Can you work these out from the model? Positions are in its coordinate system, mm. A direction names the side the tool comes from. Give positions to 0.01 mm unless a question says otherwise; leave off trailing zeros. Order: outer loops, then holes, each group sorted by start corner. A loop starts at its lowest first (then second) coordinate and runs counter-clockwise, first axis right, second up. Notation, with made-up numbers: M -15.5,33 L 21.5,33 A18 cw 21.5,60 Z; hole C 3.5,88 d10. An arc over 180 degrees is marked long. Write each question's results on one line, items separated by ' | '.
from build123d import *

# Parameters (mm, degrees)
EXTRUDE1_DEPTH              = 342.9
SKETCH2_R                   = 1.58758
SKETCH2_R_2                 = 4.826
EXTRUDE2_DEPTH              = 25
F_1_4_0_25_DIAMETER_HOLE1_D = 6.35
LPATTERN1_COUNT             = 27
LPATTERN1_PITCH             = 25.4


with BuildPart() as part:
    # Sketch1 → Extrude1 (new body, symmetric)
    with BuildSketch(Plane(origin=(0, 0, 0), x_dir=(1, 0, 0), z_dir=(0, 1, 0))):
        with BuildLine():
            Line((-12.7, 0), (-12.7, 22.225))
            ThreePointArc((-12.7, 22.225), (-11.77006403, 24.47006403), (-9.525, 25.4))
            Line((-9.525, 25.4), (9.525, 25.4))
            ThreePointArc((9.525, 25.4), (11.77006403, 24.47006403), (12.7, 22.225))
            Line((12.7, 22.225), (12.7, 0))
            Line((12.7, 0), (15.875, 0))
            Line((15.875, 0), (15.875, 22.225))
            ThreePointArc((15.875, 22.225), (14.015128061, 26.715128061), (9.525, 28.575))
            Line((9.525, 28.575), (-9.525, 28.575))
            ThreePointArc((-9.525, 28.575), (-14.015128061, 26.715128061), (-15.875, 22.225))
            Line((-15.875, 22.225), (-15.875, 0))
            Line((-15.875, 0), (-12.7, 0))
        make_face()
    extrude(amount=EXTRUDE1_DEPTH, both=True)

    # Sketch2 → Extrude2 (cut)
    with BuildSketch(Plane(origin=(0, 0, -28.575), x_dir=(-1, 0, 0), z_dir=(0, 0, -1))):
        with Locations((0, 342.9)):
            Circle(SKETCH2_R)
        with Locations((-1.905, 209.55)):
            Circle(SKETCH2_R_2)
        with Locations((-1.905, 184.15)):
            Circle(SKETCH2_R_2)
        with Locations((-1.905, -6.35)):
            Circle(SKETCH2_R_2)
        with Locations((1.905, 101.6)):
            Circle(SKETCH2_R_2)
        with Locations((-1.905, -260.35)):
            Circle(SKETCH2_R_2)
        with Locations((-1.905, -234.95)):
            Circle(SKETCH2_R_2)
        with Locations((-1.905, 19.05)):
            Circle(SKETCH2_R_2)
    extrude(amount=-EXTRUDE2_DEPTH, mode=Mode.SUBTRACT)

    # 1/4 (0.25) Diameter Hole1 (through all)
    with Locations(Plane.ZY.offset(15.875)):
        with Locations((-12.7, 330.2)):
            f_1_4_0_25_diameter_hole1 = Hole(F_1_4_0_25_DIAMETER_HOLE1_D / 2)

    # LPattern1: 1/4 (0.25) Diameter Hole1 ×27
    with Locations(*[(0, -i * LPATTERN1_PITCH, 0) for i in range(1, LPATTERN1_COUNT)]):
        add(f_1_4_0_25_diameter_hole1, mode=Mode.SUBTRACT)


solid = part.part
(1) Will these pins go through, and if not, where does the flat tip stop? P1, Ø7.5, axis at x = 1.905, y = -6.35, coming from the +Z side; P2, Ø5, axis at y = -49.5, z = -25.5, coming from the -X side.
Data:
P1: passes through | P2: stops at x = -15.83
(2) Imagine slicing it at A-A, the plane y = -294. Write out the boundary of the cut face in (x, z) (3 decimals), plus the area to 3 significant figures.
Data:
outline: M -15.875,-22.225 A6.35 ccw -9.525,-28.575 L 9.525,-28.575 A6.35 ccw 15.875,-22.225 L 15.875,0 L 12.7,0 L 12.7,-22.225 A3.175 cw 9.525,-25.4 L -9.525,-25.4 A3.175 cw -12.7,-22.225 L -12.7,0 L -15.875,0 Z | area: 249 mm2
(3) For faces 5 (the face through (-12.7, 5, -11)), 6 (the face through (0, 5, -28.575)), which set-ups out of +Z, -Z, +X, -X, +Y, -Y let a thin tool reach every point of the face, with its end or its side?
Data:
face 5: +Z, +Y, -Y | face 6: -Z, +X, -X, +Y, -Y
(4) We'd pull the mould along X, two halves only. Please class faces 1 (the face through (13, 342.9, -16)), 2 (the face through (15.875, 5, -11)), 3 (the face through (-15.875, 5, -11)), 4 (the face through (12.7, 5, -11)): +X half, -X half, draft (parallel to the pull), parting line (faces both ways), or undercut.
Data:
face 1: draft | face 2: +X half | face 3: -X half | face 4: undercut
(5) I need wall thicknesses on L1, parallel to X at y = 140.5, z = -12.75 (3 decimals); L2, parallel to Z at x = 15, y = -279; L3, parallel to Z at x = -0.5, y = -135.5 (3 decimals). Which ranges of each line are inside material? Lowest first, please. Write a range as from..to.
Data:
L1: x = -15.875..-12.7, 12.7..15.875 | L2: z = -25.44..-15.85, -9.55..0 | L3: z = -28.575..-25.4
